```python
from build123d import *

# Parameters (mm, degrees)
SKETCH_1_W          = 10
SKETCH_1_H          = 10
SKETCH_1_W_2        = 8
SKETCH_1_H_2        = 8
EXTRUDE_1_DEPTH     = 137.5
CUT_EXTRUDE_1_REACH = 139.954
SKETCH_2_R          = 2.1


with BuildPart() as part:
    # ｽｹｯﾁ1 → 押し出し-薄板1 (new body)
    with BuildSketch(Plane(origin=(0, 0, 0), x_dir=(1, 0, 0), z_dir=(0, 1, 0))):
        Rectangle(SKETCH_1_W, SKETCH_1_H)
        Rectangle(SKETCH_1_W_2, SKETCH_1_H_2, mode=Mode.SUBTRACT)
    extrude(amount=EXTRUDE_1_DEPTH)

    # ｶｯﾄ - 押し出し1: up to this face of the body (flat: up to its plane)
    cut_extrude_1_end = Plane(part.part.faces().sort_by_distance((0, 68.75, -5))[0])
    # ｽｹｯﾁ2 → ｶｯﾄ - 押し出し1 (cut, up to the picked face)
    with BuildSketch(Plane.XY.offset(5), mode=Mode.PRIVATE) as cut_extrude_1_sk1:
        with Locations((0, 132.5)):
            Circle(SKETCH_2_R)
    cut_extrude_1_tool1 = split(extrude(cut_extrude_1_sk1.sketch, amount=-CUT_EXTRUDE_1_REACH, mode=Mode.PRIVATE), bisect_by=cut_extrude_1_end, keep=Keep.BOTH, mode=Mode.PRIVATE)
    # ｽｹｯﾁ2 → ｶｯﾄ - 押し出し1 (cut, up to the picked face)
    with BuildSketch(Plane.XY.offset(5), mode=Mode.PRIVATE) as cut_extrude_1_sk2:
        with Locations(Location((0, 5, 0), (0, 0, 180))):
            Circle(SKETCH_2_R)
    cut_extrude_1_tool2 = split(extrude(cut_extrude_1_sk2.sketch, amount=-CUT_EXTRUDE_1_REACH, mode=Mode.PRIVATE), bisect_by=cut_extrude_1_end, keep=Keep.BOTH, mode=Mode.PRIVATE)
    add(cut_extrude_1_tool1.solids().sort_by(Axis((0, 132.5, 5), (0, 0, -1)))[0], mode=Mode.SUBTRACT)
    add(cut_extrude_1_tool2.solids().sort_by(Axis((0, 5, 5), (0, 0, -1)))[0], mode=Mode.SUBTRACT)


solid = part.part
```
Here's how the part is built. I have some questions about the finished solid (model axes, mm). A direction names the side the tool comes from. Give positions to 0.01 mm unless a question says otherwise; leave off trailing zeros. Order: outer loops, then holes, each group sorted by start corner. A loop starts at its lowest first (then second) coordinate and runs counter-clockwise, first axis right, second up. Notation, with made-up numbers: M 27,-5 L 37,-5 A9 cw 37,0 Z; hole C -11.5,25 d3. An arc over 180 degrees is marked long. Use a Markdown table: item, result. Add a question column.
1. I need wall thicknesses on probe 1 along Y at (x, z) = (0, -4.7); probe 2 along Z at (x, y) = (-2.5, 25.5). Which ranges of each line are inside material? Lowest first, please. Write a range as from..to.
2. If we mould it in two halves opening along Y, with no side actions, what happens to faces 3 (the flat face through (-4.5, 0, -0.1)), 4 (the cylindrical face through (0.46, 7.05, -4.49)), 5 (the flat face through (0, 68, -5))? For each: +Y half, -Y half, draft (parallel to the pull), parting line (faces both ways), or undercut.
3. Suppose I cut it at C-C (z = -2.25). List the corners of the cut face in (x, y) for me, and give its area (3 significant figures).
4. Suppose I cut it at B-B (x = 0). List the corners of the cut face in (y, z) for me.
5. On a 3-axis mill with a long thin cutter (end or side, diameter ignored), from which of +Z, -Z, +X, -X, +Y, -Y can I reach the whole of each face in a straight line? I mean faces 1 (the flat face through (0, 68, -4)), 2 (the flat face through (-5, 68, 0)). Say none if no direction works.
6. Suppose I cut it at A-A (y = 5). List the corners of the cut face in (x, z) for me, and give its area (3 significant figures).
7. Suppose I cut it at D-D (y = 48). List the corners of the cut face in (x, z) for me.
Results list:
| question | item | result |
|---|---|---|
| 1 | probe 1 | y = 0..2.9, 7.1..130.4, 134.6..137.5 |
| 1 | probe 2 | z = -5..-4, 4..5 |
| 2 | face 3 | -Y half |
| 2 | face 4 | undercut |
| 2 | face 5 | draft |
| 3 | outline | M -5,0 L -4,0 L -4,137.5 L -5,137.5 Z; M 4,0 L 5,0 L 5,137.5 L 4,137.5 Z |
| 3 | area | 275 mm² |
| 4 | outline | M 0,-5 L 2.9,-5 L 2.9,-4 L 0,-4 Z; M 0,4 L 2.9,4 L 2.9,5 L 0,5 Z; M 7.1,-5 L 130.4,-5 L 130.4,-4 L 7.1,-4 Z; M 7.1,4 L 130.4,4 L 130.4,5 L 7.1,5 Z; M 134.6,-5 L 137.5,-5 L 137.5,-4 L 134.6,-4 Z; M 134.6,4 L 137.5,4 L 137.5,5 L 134.6,5 Z |
| 5 | face 1 | +Y, -Y |
| 5 | face 2 | +Z, -Z, -X, +Y, -Y |
| 6 | outline | M -5,-5 L -2.1,-5 L -2.1,-4 L -4,-4 L -4,4 L -2.1,4 L -2.1,5 L -5,5 Z; M 2.1,-5 L 5,-5 L 5,5 L 2.1,5 L 2.1,4 L 4,4 L 4,-4 L 2.1,-4 Z |
| 6 | area | 27.6 mm² |
| 7 | outline | M -5,-5 L 5,-5 L 5,5 L -5,5 Z; hole M -4,-4 L 4,-4 L 4,4 L -4,4 Z |
